Check sheet for the modelled part. Datum: model origin and axes. Units: mm. A direction names the side the tool comes from. Round coordinates to 2 decimals unless told otherwise and drop trailing zeros. Order: outer loops, then holes, each group sorted by start corner. A loop starts at its lowest first (then second) coordinate and runs counter-clockwise, first axis right, second up. Notation, with made-up numbers: (-2, 71) -> (9, 71) arc R11 cw to (9, 88) -> close; hole circle Ø7 at (15, 35.5). An arc over 180 degrees is marked (long way). Answer in a Markdown table with one row per item. Add a question column.
1. Sectioned sample at C-C, the plane z = 13. Record the boundary of the cut face in (x, y).
2. Material ranges on L1, parallel to X at y = -12, z = 2.75; L2, parallel to Z at x = -11, y = 15.5; L3, parallel to Z at x = -27, y = -17, recorded low to high. Write a range as from..to.
3. Depth check by flat-ended pin: P1, Ø8.5, axis at x = -2, z = 4.5, coming from the -Y side; P2, Ø3, axis at x = 38, z = 5.5, coming from the -Y side; P3, Ø8, axis at y = 4, z = 6.5, coming from the -X side. Enter the tip coordinate at first touch or a pass-through.
4. Sectioned sample at D-D, the plane x = -38. Record the boundary of the cut face in (y, z), then the cut area to 3 significant figures.
5. Access from +Z, -Z, +X, -X, +Y, -Y to the whole of each face (thin tool, end or side, straight path). Record for faces 1 (the flat face through (-19.6, -29.4, 2.5)), 2 (the flat face through (0, 10.5, 7)), 3 (the flat face through (0, 13, 15)).
6. Draft check along X on faces 4 (the cylindrical face through (0.436, 22.496, 2.465)), 5 (the cylindrical face through (-0.176, 1.503, 7.395)), 6 (the flat face through (-1, -7, 0)). Enter one of: +X half, -X half, draft (parallel to the pull), parting line (faces both ways), or undercut.
7. Sectioned sample at A-A, the plane x = 0. Record the boundary of the cut face in (y, z), then the cut area to 3 significant figures.
8. Sectioned sample at B-B, the plane y = 7.5. Record the boundary of the cut face in (x, z).
```python
from build123d import *

# Parameters (mm, degrees)
BOSS_EXTRUDE1_DEPTH  = 5
M3_CLEARANCE_HOLE1_D = 3.8
BOSS_EXTRUDE3_START  = 5
SKETCH2_6_R          = 12.5
BOSS_EXTRUDE3_DEPTH  = 10
FILLET1_R            = 2


with BuildPart() as part:
    # Sketch2 → Boss-Extrude1 (new body)
    with BuildSketch(Plane.XY):
        with BuildLine():
            Line((6.578363356, -21.516857009), (32.24208854, -37.05304733))
            Line((32.24208854, -37.05304733), (47.778278861, -11.389322146))
            Line((47.778278861, -11.389322146), (22.114553677, 4.146868175))
            ThreePointArc((22.114553677, 4.146868175), (0, 22.5), (-22.114553677, 4.146868175))
            Line((-22.114553677, 4.146868175), (-47.778278861, -11.389322146))
            Line((-47.778278861, -11.389322146), (-32.24208854, -37.05304733))
            Line((-32.24208854, -37.05304733), (-6.578363356, -21.516857009))
            ThreePointArc((-6.578363356, -21.516857009), (0, -22.5), (6.578363356, -21.516857009))
        make_face()
        with BuildLine():
            Line((5.196152423, 10.5), (-5.196152423, 10.5))
            ThreePointArc((-5.196152423, 10.5), (0, 1.5), (5.196152423, 10.5))
        make_face(mode=Mode.SUBTRACT)
    extrude(amount=BOSS_EXTRUDE1_DEPTH)

    # M3 Clearance Hole1 (through all)
    with Locations(Plane.XY.offset(5)):
        with Locations((-40.911626277, -13.077244623), (-23.802476154, -2.719784409), (-13.44501594, -19.828934532), (-30.554166063, -30.186394746), (13.44501594, -19.828934532), (23.802476154, -2.719784409), (40.911626277, -13.077244623), (30.554166063, -30.186394746)):
            Hole(M3_CLEARANCE_HOLE1_D / 2)

    # Sketch2<6> → Boss-Extrude3 (add)
    with BuildSketch(Plane.XY.offset(BOSS_EXTRUDE3_START)):
        with Locations((0, 7.5)):
            Circle(SKETCH2_6_R)
        with BuildLine():
            ThreePointArc((-5.196152423, 10.5), (0, 1.5), (5.196152423, 10.5))
            Line((5.196152423, 10.5), (-5.196152423, 10.5))
        make_face(mode=Mode.SUBTRACT)
    extrude(amount=BOSS_EXTRUDE3_DEPTH)

    # Fillet1
    fillet1_edges = [part.edges().sort_by_distance(p)[0] for p in [
        (-12.5, 7.5, 5),
    ]]
    fillet(fillet1_edges, radius=FILLET1_R)


solid = part.part
```
Answer key:
| question | item | result |
|---|---|---|
| 1 | outline | circle Ø25 at (0, 7.5); hole (-5.2, 10.5) arc R6 ccw (long way) to (5.2, 10.5) -> close |
| 2 | L1 | x = -47.41..-42.48, -39.35..39.35, 42.48..47.41 |
| 2 | L2 | z = 0..5.21 |
| 2 | L3 | z = 0..5 |
| 3 | P1 | stops at y = -22.5 |
| 3 | P2 | stops at y = -29.88 |
| 3 | P3 | stops at x = -28.48 |
| 4 | outline | (-27.54, 0) -> (-5.47, 0) -> (-5.47, 5) -> (-27.54, 5) -> close |
| 4 | area | 110 mm² |
| 5 | face 1 | +Z, -Z, -Y |
| 5 | face 2 | +Z, -Z |
| 5 | face 3 | +Z, +X, -X, +Y, -Y |
| 6 | face 4 | parting line |
| 6 | face 5 | undercut |
| 6 | face 6 | draft |
| 7 | outline | (-22.5, 0) -> (1.5, 0) -> (1.5, 15) -> (-5, 15) -> (-5, 7) arc R2 cw to (-7, 5) -> (-22.5, 5) -> close; (10.5, 0) -> (22.5, 0) -> (22.5, 5) -> (22, 5) arc R2 cw to (20, 7) -> (20, 15) -> (10.5, 15) -> close |
| 7 | area | 342 mm² |
| 8 | outline | (-21.21, 0) -> (-6, 0) -> (-6, 15) -> (-12.5, 15) -> (-12.5, 7) arc R2 cw to (-14.5, 5) -> (-21.21, 5) -> close; (6, 0) -> (21.21, 0) -> (21.21, 5) -> (14.5, 5) arc R2 cw to (12.5, 7) -> (12.5, 15) -> (6, 15) -> close |
